The model under review builds one solid part; all positions refer to its coordinate system, in mm. A direction names the side the tool comes from. Round coordinates to 2 decimals unless told otherwise and drop trailing zeros. Order: outer loops, then holes, each group sorted by start corner. A loop starts at its lowest first (then second) coordinate and runs counter-clockwise, first axis right, second up. Notation, with made-up numbers: (-11, -27.5) - (40, -27.5) arc R14 ccw to (40, -18.5) - close; hole circle Ø9 at (53.25, -8.5). An arc over 180 degrees is marked (long way). One line per question, with ' | ' between items. Start each with the question number.
Item 1: Insertion check: pin 1 Ø1.8 at (x, z) = (0.5, 9) entering from -Y; pin 2 Ø1.3 at (x, z) = (-0.5, -33) entering from -Y; pin 3 Ø3 at (x, z) = (9.1, -9) entering from -Y; pin 4 Ø1.7 at (x, z) = (-8, 23) entering from +Y. Each pin has a flat end and moves straight along its axis. Give the tip position at first contact, or say it passes through.
Item 2: Draft analysis for pull direction Z (two halves, no side actions). For faces 4 (the face through (9, 6, 21.05)), 5 (the face through (-27.07, 4.06, 43.5)), 6 (the face through (-28.5, 4, 1)), state which applies: +Z half, -Z half, draft (parallel to the pull), parting line (faces both ways), or undercut.
Item 3: Add section A-A on z = -34. State the section outline as (x, y) points.
Item 4: For L1, parallel to Z at x = 0, y = 6.95; L2, parallel to Z at x = 0, y = 5.65; L3, parallel to X at y = 2.2, z = 23.9, list the stretches that pass through material, from the lowest coordinate up. Write a range as [from, to].
Item 5: Tool access review of faces 1 (the face through (-11.58, 5.535, -7.595)), 2 (the face through (-0.249, 7.26, -32.877)), 3 (the face through (1, 6.5, -35)): name each direction out of +Z, -Z, +X, -X, +Y, -Y from which nothing blocks a thin tool from reaching the whole face with its end or side.
Item 6: Add section B-B on y = 4. State how many separate pieces and enclosed holes the cut face has, and give its area (3 significant figures).
from build123d import *

# Parameters (mm, degrees)
SKETCH_1_W          = 57
SKETCH_1_H          = 90
SKETCH_1_R          = 5
SKETCH_1_R_2        = 1.65
EXTRUDE_1_DEPTH     = 8
CUT_EXTRUDE_1_DEPTH = 5
SKETCH_3_R          = 3
CUT_EXTRUDE_2_DEPTH = 5
FILLET_1_R          = 5
SKETCH_4_R          = 1.15
CUT_EXTRUDE_3_DEPTH = 9
SKETCH_5_R          = 2.15
CUT_EXTRUDE_4_DEPTH = 6.5


with BuildPart() as part:
    # 草图1 → 凸台-拉伸1 (new body)
    with BuildSketch(Plane(origin=(0, 0, 0), x_dir=(1, 0, 0), z_dir=(0, 1, 0))):
        Rectangle(SKETCH_1_W, SKETCH_1_H)
        Circle(SKETCH_1_R, mode=Mode.SUBTRACT)
        with Locations((0, 7.954951288)):
            Circle(SKETCH_1_R_2, mode=Mode.SUBTRACT)
        with Locations((7.954951288, 0)):
            Circle(SKETCH_1_R_2, mode=Mode.SUBTRACT)
        with Locations((0, -7.954951288)):
            Circle(SKETCH_1_R_2, mode=Mode.SUBTRACT)
        with Locations((-7.954951288, 0)):
            Circle(SKETCH_1_R_2, mode=Mode.SUBTRACT)
        with Locations((9.1, 9)):
            Circle(SKETCH_1_R_2, mode=Mode.SUBTRACT)
        with Locations((-9.1, 9)):
            Circle(SKETCH_1_R_2, mode=Mode.SUBTRACT)
        with Locations((-9.1, -23.9)):
            Circle(SKETCH_1_R_2, mode=Mode.SUBTRACT)
        with Locations((9.1, -23.9)):
            Circle(SKETCH_1_R_2, mode=Mode.SUBTRACT)
    extrude(amount=EXTRUDE_1_DEPTH)

    # 草图2 → 切除-拉伸1 (cut)
    with BuildSketch(Plane(origin=(0, 8, 0), x_dir=(1, 0, 0), z_dir=(0, 1, 0))):
        Polygon((-7.454551733, 11.85), (-10.745448267, 11.85), (-12.390896534, 9), (-10.745448267, 6.15), (-7.454551733, 6.15), (-5.809103466, 9), align=None)
        Polygon((10.745448267, 11.85), (7.454551733, 11.85), (5.809103466, 9), (7.454551733, 6.15), (10.745448267, 6.15), (12.390896534, 9), align=None)
        Polygon((10.745448267, -21.05), (7.454551733, -21.05), (5.809103466, -23.9), (7.454551733, -26.75), (10.745448267, -26.75), (12.390896534, -23.9), align=None)
        Polygon((-10.745448267, -21.05), (-12.390896534, -23.9), (-10.745448267, -26.75), (-7.454551733, -26.75), (-5.809103466, -23.9), (-7.454551733, -21.05), align=None)
    extrude(amount=-CUT_EXTRUDE_1_DEPTH, mode=Mode.SUBTRACT)

    # 草图3 → 切除-拉伸2 (cut)
    with BuildSketch(Plane.XZ):
        with Locations((0, 7.954951288)):
            Circle(SKETCH_3_R)
        with Locations((7.954951288, 0)):
            Circle(SKETCH_3_R)
        with Locations((0, -7.954951288)):
            Circle(SKETCH_3_R)
        with Locations((-7.954951288, 0)):
            Circle(SKETCH_3_R)
    extrude(amount=-CUT_EXTRUDE_2_DEPTH, mode=Mode.SUBTRACT)

    # 圆角1
    fillet_1_edges = [part.edges().sort_by_distance(p)[0] for p in [
        (28.5, 4, 45),
        (-28.5, 4, 45),
        (-28.5, 4, -45),
        (28.5, 4, -45),
    ]]
    fillet(fillet_1_edges, radius=FILLET_1_R)

    # 草图4 → 切除-拉伸3 (cut, through all)
    with BuildSketch(Plane(origin=(0, 8, 0), x_dir=(1, 0, 0), z_dir=(0, 1, 0))):
        with Locations((0, 34)):
            Circle(SKETCH_4_R)
    extrude(amount=-CUT_EXTRUDE_3_DEPTH, mode=Mode.SUBTRACT)

    # 草图5 → 切除-拉伸4 (cut)
    with BuildSketch(Plane.XZ):
        with Locations((0, -34)):
            Circle(SKETCH_5_R)
    extrude(amount=-CUT_EXTRUDE_4_DEPTH, mode=Mode.SUBTRACT)


solid = part.part
Determined:
1) pin 1: y = 5 | pin 2: y = 6.5 | pin 3: through | pin 4: y = 3
2) face 4: undercut | face 5: +Z half | face 6: draft
3) outline: (-28.5, 0) - (-2.15, 0) - (-2.15, 6.5) - (-1.15, 6.5) - (-1.15, 8) - (-28.5, 8) - close; (1.15, 6.5) - (2.15, 6.5) - (2.15, 0) - (28.5, 0) - (28.5, 8) - (1.15, 8) - close
4) L1: [-45, -35.15], [-32.85, -9.6], [-6.3, -5], [5, 6.3], [9.6, 45] | L2: [-45, -36.15], [-31.85, -9.6], [-6.3, -5], [5, 6.3], [9.6, 45] | L3: [-28.5, -10.75], [-7.45, 7.45], [10.75, 28.5]
5) face 1: +Y | face 2: +Y, -Y | face 3: -Y
6) separate pieces: 1 | enclosed holes: 6 | area: 4,790 mm2
